Autodesk Inventor part; units mm, degrees
ref_plane "YZ Plane" through (0, 0, 0) normal (1, 0, 0) x (0, 1, 0)
ref_plane "XZ Plane" through (0, 0, 0) normal (0, 1, 0) x (-1, 0, 0)
ref_plane "XY Plane" through (0, 0, 0) normal (0, 0, 1) x (1, 0, 0)
sketch "Sketch1" plane through (0, 0, 0) normal (0, 0, 1) x (1, 0, 0)
  circle A0 centre (0, 0) radius 27.7794
  line L0 (-15.1761, -27.7794) -> (15.5731, -27.7794)
  circle A1 centre (0, 0) radius 26.4642
  dimension "d13" = 55.5588
  dimension "SupportThickness" = 1.3152
extrude "Extrusion1" add sketch "Sketch1" along normal blind 1.3152 contours A0 | A1
extrude "Extrusion3" add sketch "Sketch1" against normal blind 8.6848
equation "\"d13\" = 1.1 * CrucibleOuterDiameter"
equation "\"d1\" = SupportThickness"
equation "\"d15\" = SupportHeight - SupportThickness"
equation "\"CrucibleOuterDiameter\" = 50.508"
equation "\"SupportHeight\" = 10"
properties part number "crucible_support"
Design review of the part built by this model. Coordinates are the model's own, in mm. Coordinates: 2 decimals unless noted, no trailing zeros. Loops run counter-clockwise (first coordinate to the right, second up) from the corner with the lowest first, then second, coordinate; pieces in that order, holes last. Notation, with made-up numbers: (59, 75) -> (104, 75) arc R22 cw to (104, 105) -> close; hole circle Ø4 at (55, -38.5). An arc over 180 degrees is marked (long way). Use a Markdown table: item, result. Add a question column.
Item 1: We need section A-A, the plane x = 0. Write out the cut boundary in (y, z), and give its area (3 significant figures).
Item 2: Wall thickness on L1, parallel to Y at x = 0, z = -6; L2, parallel to Y at x = -5, z = -8; L3, parallel to Z at x = 3.5, y = -22: over which ranges is each line inside the solid? List them lowest first. Write a range as from..to.
Item 3: We need section C-C, the plane z = -2.25. Write out the cut boundary in (x, y), and give its area (3 significant figures).
Item 4: Clearance check with flat-ended pins moving along their axes: P1, Ø1, axis at x = -18.5, z = 0, coming from the +Y side; P2, Ø6, axis at x = 18, z = -4, coming from the +Y side; P3, Ø6, axis at x = -6, z = -5.5, coming from the +Y side. State where each tip first meets the part, or that it passes through.
Item 5: The part is to be moulded in two halves that separate along X. For faces 1 (the flat face through (25, -10, -8.685)), 2 (the cylindrical face through (-22.045, -16.903, -3.615)), 3 (the cylindrical face through (-5.737, -25.835, -4.282)), 4 (the flat face through (0, 0, 0)), say which applies: +X half, -X half, draft (parallel to the pull), parting line (faces both ways), or undercut.
Numbers:
| question | item | result |
|---|---|---|
| 1 | outline | (-27.78, -8.68) -> (-26.46, -8.68) -> (-26.46, 0) -> (26.46, 0) -> (26.46, -8.68) -> (27.78, -8.68) -> (27.78, 1.32) -> (-27.78, 1.32) -> close |
| 1 | area | 95.9 mm^2 |
| 2 | L1 | y = -27.78..-26.46, 26.46..27.78 |
| 2 | L2 | y = -27.33..-25.99, 25.99..27.33 |
| 2 | L3 | z = 0..1.32 |
| 3 | outline | circle Ø55.56 at (0, 0); hole circle Ø52.93 at (0, 0) |
| 3 | area | 224 mm^2 |
| 4 | P1 | stops at y = 21.16 |
| 4 | P2 | stops at y = 23.38 |
| 4 | P3 | stops at y = 27.62 |
| 5 | face 1 | draft |
| 5 | face 2 | parting line |
| 5 | face 3 | undercut |
| 5 | face 4 | undercut |
